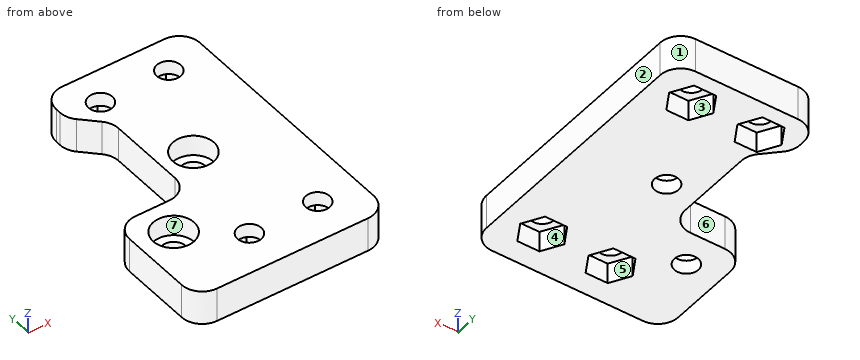
from build123d import *

# Parameters (mm, degrees)
SKETCH2_R           = 1.75
BOSS_EXTRUDE1_DEPTH = 5
SKETCH3_R           = 3
CUT_EXTRUDE1_DEPTH  = 3
FILLET1_R           = 3
CUT_EXTRUDE2_DEPTH  = 3


with BuildPart() as part:
    # Sketch2 → Boss-Extrude1 (new body)
    with BuildSketch(Plane.XY):
        Polygon((11, -21), (11, 20), (-10, 20), (-10, 15), (-6.1, 11.1), (-6.1, -4.5), (-17.1, -4.5), (-17.1, -21), align=None)
        with Locations((-1.5, 1.1)):
            Circle(SKETCH2_R, mode=Mode.SUBTRACT)
        with Locations((-12.1, -9.5)):
            Circle(SKETCH2_R, mode=Mode.SUBTRACT)
        with Locations((-5, 15)):
            Circle(SKETCH2_R, mode=Mode.SUBTRACT)
        with Locations((-5, -15)):
            Circle(SKETCH2_R, mode=Mode.SUBTRACT)
        with Locations((5, 15)):
            Circle(SKETCH2_R, mode=Mode.SUBTRACT)
        with Locations((5, -15)):
            Circle(SKETCH2_R, mode=Mode.SUBTRACT)
    extrude(amount=BOSS_EXTRUDE1_DEPTH)

    # Sketch3 → Cut-Extrude1 (cut)
    with BuildSketch(Plane.XY.offset(5)):
        with Locations((-1.5, 1.1)):
            Circle(SKETCH3_R)
        with Locations((-12.1, -9.5)):
            Circle(SKETCH3_R)
    extrude(amount=-CUT_EXTRUDE1_DEPTH, mode=Mode.SUBTRACT)

    # Fillet1
    fillet1_edges = [part.edges().sort_by_distance(p)[0] for p in [
        (-6.1, -4.5, 2.5),
        (-6.1, 11.1, 2.5),
        (-10, 15, 2.5),
        (-10, 20, 2.5),
        (11, 20, 2.5),
        (11, -21, 2.5),
        (-17.1, -21, 2.5),
        (-17.1, -4.5, 2.5),
    ]]
    fillet(fillet1_edges, radius=FILLET1_R)

    # Sketch4 → Cut-Extrude2 (cut)
    with BuildSketch(Plane(origin=(0, 0, 0), x_dir=(-1, 0, 0), z_dir=(0, 0, -1))):
        Polygon((-3.383419246, 12.2), (-1.766838493, 15), (-3.383419246, 17.8), (-6.616580754, 17.8), (-8.233161507, 15), (-6.616580754, 12.2), align=None)
        Polygon((6.616580754, 12.2), (8.233161507, 15), (6.616580754, 17.8), (3.383419246, 17.8), (1.766838493, 15), (3.383419246, 12.2), align=None)
        Polygon((-3.383419246, -17.8), (-1.766838493, -15), (-3.383419246, -12.2), (-6.616580754, -12.2), (-8.233161507, -15), (-6.616580754, -17.8), align=None)
        Polygon((6.616580754, -17.8), (8.233161507, -15), (6.616580754, -12.2), (3.383419246, -12.2), (1.766838493, -15), (3.383419246, -17.8), align=None)
    extrude(amount=-CUT_EXTRUDE2_DEPTH, mode=Mode.SUBTRACT)


solid = part.part
Work out the finished part from the listing and answer in its coordinate system (mm). Face numbers are marked on the shaded views. A direction names the side the tool comes from. Give positions to 0.01 mm unless a question says otherwise; leave off trailing zeros. Order: outer loops, then holes, each group sorted by start corner. A loop starts at its lowest first (then second) coordinate and runs counter-clockwise, first axis right, second up. Notation, with made-up numbers: (-34, 4) -> (-28, 4) arc R11 ccw to (-28, 25) -> close; hole circle Ø1 at (2.5, -32.75). An arc over 180 degrees is marked (long way). Answer as a JSON object with one key per item and string values. Group by question number.
1. The mould has two halves that part along Y. Classify the marked faces 1, 2, 3 and 4: released by +Y, released by -Y, zero draft, split by the parting line, or undercut.
2. Section A-A on x = 5 is taken. Determine the outline of the cut face in (y, z).
3. Section D-D on x = 1 is taken. Determine the outline of the cut face in (y, z), plus the area to 3 significant figures.
4. A tool of negligible diameter and unlimited length cuts with its end or side. For the marked faces 5, 6 and 7, from which of +Z, -Z, +X, -X, +Y, -Y can it reach the whole face along a straight path? Write none if from no direction.
5. Consider line 1 along Y through (x, z) = (4.75, 2.1); line 2 along X through (y, z) = (-15, 3.7); line 3 along Y through (x, z) = (-5, 3.5). Determine where each line is inside the solid, lowest interval first. Write a range as [from, to].
6. Flat-ended cylindrical pins translate along their axes: pin 1 Ø1.7 at (x, y) = (5, -16) entering from -Z; pin 2 Ø5 at (x, y) = (-12.1, -9.5) entering from +Z; pin 3 Ø0.6 at (y, z) = (16.5, 3.5) entering from -X. Find the tip coordinate at first contact, or state that the pin passes through.
7. Section C-C on x = -12.5 is taken. Determine the outline of the cut face in (y, z), plus the area to 3 significant figures.
8. Section B-B on z = 4.4 is taken. Determine the outline of the cut face in (x, y), plus the area to 3 significant figures.
Result sheet:
{
 "1": {"face 1": "released by +Y", "face 2": "zero draft", "face 3": "undercut", "face 4": "undercut"},
 "2": {"outline": "(-21, 0) -> (-17.8, 0) -> (-17.8, 3) -> (-16.75, 3) -> (-16.75, 5) -> (-21, 5) -> close; (-13.25, 3) -> (-12.2, 3) -> (-12.2, 0) -> (12.2, 0) -> (12.2, 3) -> (13.25, 3) -> (13.25, 5) -> (-13.25, 5) -> close; (16.75, 3) -> (17.8, 3) -> (17.8, 0) -> (20, 0) -> (20, 5) -> (16.75, 5) -> close"},
 "3": {"outline": "(-21, 0) -> (20, 0) -> (20, 5) -> (2.76, 5) -> (2.76, 2) -> (-0.56, 2) -> (-0.56, 5) -> (-21, 5) -> close", "area": "195 mm^2"},
 "4": {"face 5": "-Z", "face 6": "+Z, -Z, -X", "face 7": "+Z"},
 "5": {"line 1": "y = [-21, -17.8], [-12.2, 12.2], [17.8, 20]", "line 2": "x = [-17.1, -6.75], [-3.25, 3.25], [6.75, 11]", "line 3": "y = [-21, -16.75], [-13.25, 13.25], [16.75, 20]"},
 "6": {"pin 1": "stops at z = 3", "pin 2": "stops at z = 2", "pin 3": "stops at x = -10"},
 "7": {"outline": "(-21, 0) -> (-11.2, 0) -> (-11.2, 2) -> (-12.47, 2) -> (-12.47, 5) -> (-21, 5) -> close; (-7.8, 0) -> (-4.5, 0) -> (-4.5, 5) -> (-6.53, 5) -> (-6.53, 2) -> (-7.8, 2) -> close", "area": "57.8 mm^2"},
 "8": {"outline": "(-17.1, -18) arc R3 ccw to (-14.1, -21) -> (8, -21) arc R3 ccw to (11, -18) -> (11, 17) arc R3 ccw to (8, 20) -> (-7, 20) arc R3 ccw to (-10, 17) -> (-10, 16.24) arc R3 ccw to (-9.12, 14.12) -> (-6.98, 11.98) arc R3 cw to (-6.1, 9.86) -> (-6.1, -1.5) arc R3 cw to (-9.1, -4.5) -> (-14.1, -4.5) arc R3 ccw to (-17.1, -7.5) -> close; hole circle Ø6 at (-12.1, -9.5); hole circle Ø3.5 at (-5, -15); hole circle Ø3.5 at (-5, 15); hole circle Ø6 at (-1.5, 1.1); hole circle Ø3.5 at (5, -15); hole circle Ø3.5 at (5, 15)", "area": "807 mm^2"}
}
